Geometry check sheet. Reference: the model listing, model coordinates, mm. Round coordinates to 2 decimals unless told otherwise and drop trailing zeros. Write each loop counter-clockwise with the first axis right and the second up, starting at its lowest first coordinate (ties: lowest second). Pieces come first, ordered by that corner, then holes.
Autodesk Inventor part; units mm, degrees
ref_plane "YZ Plane" through (0, 0, 0) normal (1, 0, 0) x (0, 1, 0)
ref_plane "XZ Plane" through (0, 0, 0) normal (0, 1, 0) x (-1, 0, 0)
ref_plane "XY Plane" through (0, 0, 0) normal (0, 0, 1) x (1, 0, 0)
sketch "Sketch1" plane through (0, 0, 0) normal (0, 0, 1) x (1, 0, 0)
  circle A0 centre (0, 0) radius 24
  circle A1 centre (0, 0) radius 7.55
  dimension "d0" = 48
  dimension "d1" = 15.1
extrude "Extrusion1" add sketch "Sketch1" along normal blind 0.32
sketch "Sketch2" plane through (0, 0, 0) normal (0, 0, -1) x (-1, 0, 0)
  circle A0 centre (-16.5319, -11.256) radius 2.05
  circle A1 centre (-19.649, 3.7306) radius 2.05
  circle A2 centre (-17.0544, -2.5903) radius 1.65
  circle A3 centre (-6.284, -16.0647) radius 1.65
  circle A4 centre (-6.284, -16.0647) radius 1.65
  circle A5 centre (-6.284, -16.0647) radius 2.125
  circle A6 centre (10.7704, -13.4744) radius 2.125
  circle A7 centre (17.0544, 2.5903) radius 2.125
  circle A8 centre (6.284, 16.0647) radius 2.125
  circle A9 centre (-10.7704, 13.4744) radius 2.125
  circle A10 centre (-17.0544, -2.5903) radius 2.125
  point P0 (0, 0)
  dimension "d4" = 4.25
  dimension "d7" = 360
extrude "Extrusion2" cut sketch "Sketch2" against normal through all contours A2 | A3 | A5 | A6 | A7 | A8 | A9 | A10
properties part number "spool_spacer"
1. Section check B-B (y = 2). Record the cut outline in (x, z), plus the area to 3 significant figures.
2. Section check A-A (x = 0). Record the cut outline in (y, z).
3. Release check for a two-part mould opening along X. For faces 1 (the face through (-23.977, -1.055, 0.158)), 2 (the face through (5, 6, 0.32)), 3 (the face through (-15.368, 1.297, 0.158)) record: +X half, -X half, draft (parallel to the pull), parting line (faces both ways), or undercut.
4. Section check C-C (z = 0.2). Record the cut outline in (x, y) (3 decimals), plus the area to 3 significant figures.
5. Scan lines: line 1 along Y through (x, z) = (0, 0.25); line 2 along X through (y, z) = (3.5, 0.1); line 3 along Y through (x, z) = (-6, 0.1). Record each from-to range of solid material in increasing order.
6. Section check D-D (x = 18.5). Record the cut outline in (y, z).
Results below:
1. outline: (-23.92, 0) - (-19.1, 0) - (-19.1, 0.32) - (-23.92, 0.32) - close; (-15.01, 0) - (-7.28, 0) - (-7.28, 0.32) - (-15.01, 0.32) - close; (7.28, 0) - (23.92, 0) - (23.92, 0.32) - (7.28, 0.32) - close
1. area: 9.34 mm2
2. outline: (-24, 0) - (-7.55, 0) - (-7.55, 0.32) - (-24, 0.32) - close; (7.55, 0) - (24, 0) - (24, 0.32) - (7.55, 0.32) - close
3. face 1: parting line
3. face 2: draft
3. face 3: undercut
4. outline: circle Ø48 at (0, 0); hole circle Ø4.25 at (-17.054, 2.59); hole circle Ø4.25 at (-10.77, -13.474); hole circle Ø4.25 at (-6.284, 16.065); hole circle Ø15.1 at (0, 0); hole circle Ø4.25 at (6.284, -16.065); hole circle Ø4.25 at (10.77, 13.474); hole circle Ø4.25 at (17.054, -2.59)
4. area: 1,550 mm2
5. line 1: y = -24 to -7.55, 7.55 to 24
5. line 2: x = -23.74 to -18.97, -15.13 to -6.69, 6.69 to 23.74
5. line 3: y = -23.24 to -4.58, 4.58 to 13.96, 18.17 to 23.24
6. outline: (-15.29, 0) - (-4.15, 0) - (-4.15, 0.32) - (-15.29, 0.32) - close; (-1.03, 0) - (15.29, 0) - (15.29, 0.32) - (-1.03, 0.32) - close
